from build123d import *

# Parameters (mm, degrees)
SKETCH1_R           = 4
BOSS_EXTRUDE1_DEPTH = 160
CUT_EXTRUDE1_DEPTH  = 7.5
SKETCH3_R           = 4
SKETCH3_R_2         = 3.5
CUT_EXTRUDE2_DEPTH  = 1


with BuildPart() as part:
    # Sketch1 → Boss-Extrude1 (new body)
    with BuildSketch(Plane.XY):
        Circle(SKETCH1_R)
    extrude(amount=BOSS_EXTRUDE1_DEPTH)

    # Sketch2 → Cut-Extrude1 (cut)
    with BuildSketch(Plane.XY.offset(160)):
        with BuildLine():
            Line((3.122498999, 2.5), (-3.122498999, 2.5))
            ThreePointArc((-3.122498999, 2.5), (0, 4), (3.122498999, 2.5))
        make_face()
    extrude(amount=-CUT_EXTRUDE1_DEPTH, mode=Mode.SUBTRACT)

    # Sketch3 → Cut-Extrude2 (cut)
    with BuildSketch(Plane.XY.offset(158.75)):
        Circle(SKETCH3_R)
        Circle(SKETCH3_R_2, mode=Mode.SUBTRACT)
    extrude(amount=-CUT_EXTRUDE2_DEPTH, mode=Mode.SUBTRACT)


solid = part.part
Geometry check sheet. Reference: the model listing, model coordinates, mm. A direction names the side the tool comes from. Give positions to 0.01 mm unless a question says otherwise; leave off trailing zeros. Order: outer loops, then holes, each group sorted by start corner. A loop starts at its lowest first (then second) coordinate and runs counter-clockwise, first axis right, second up. Notation, with made-up numbers: (-34, 60.25) - (20, 60.25) arc R13 ccw to (20, 65.25) - close; hole circle Ø1 at (-12, 37.25). An arc over 180 degrees is marked (long way). Answer as a JSON object with one key per item and string values.
(1) Cross-section at B-B (x = -1). Record the cut outline in (y, z).
Report:
{"outline": "(-3.87, 0) - (3.87, 0) - (3.87, 152.5) - (2.5, 152.5) - (2.5, 160) - (-3.87, 160) - (-3.87, 158.75) - (-3.35, 158.75) - (-3.35, 157.75) - (-3.87, 157.75) - close"}
(2) Tool access check on faces 1 (the flat face through (0, 2.5, 156)), 2 (the cylindrical face through (0, -4, 159)), 3 (the cylindrical face through (-0.1, -3.5, 158.3)). Record the directions out of +Z, -Z, +X, -X, +Y, -Y that give a thin tool (end or side, any length) a straight path to the whole face; none if there is none.
Report:
{"face 1": "+Z, +X, -X, +Y", "face 2": "+Z, -Z", "face 3": "none"}
(3) Draft check along Z on faces 4 (the cylindrical face through (-0.867, -3.905, 77.771)), 5 (the flat face through (-0.61, -3.62, 158.75)), 6 (the flat face through (0, -1, 160)). Enter one of: released by +Z, released by -Z, zero draft, split by the parting line, or undercut.
Report:
{"face 4": "zero draft", "face 5": "undercut", "face 6": "released by +Z"}
(4) Cross-section at A-A (z = 145.5). Record the cut outline in (x, y).
Report:
{"outline": "circle Ø8 at (0, 0)"}
(5) Depth check by flat-ended pin: pin 1 Ø3 at (x, z) = (0, 155) entering from +Y; pin 2 Ø1 at (x, z) = (2, 131.5) entering from -Y. Enter the tip coordinate at first touch or a pass-through.
Report:
{"pin 1": "y = 2.5", "pin 2": "y = -3.71"}
(6) Material ranges on line 1 (Z direction, x = -3.5, y = -1.5); line 2 (Y direction, x = -2.5, z = 121.5); line 3 (Y direction, x = -0.25, z = 121), recorded low to high.
Report:
{"line 1": "0 to 157.75, 158.75 to 160", "line 2": "-3.12 to 3.12", "line 3": "-3.99 to 3.99"}
